CAD build for the part. Positions are in the model's coordinates, mm. Give positions to 0.01 mm unless a question says otherwise; leave off trailing zeros. Loops run counter-clockwise (first coordinate to the right, second up) from the corner with the lowest first, then second, coordinate; pieces in that order, holes last. Notation, with made-up numbers: (69.5, 38) -> (95.5, 38) arc R33 cw to (95.5, 75) -> close; hole circle Ø4 at (8.25, 86). An arc over 180 degrees is marked (long way). Use one line per item in the form item = value.
```python
from build123d import *

# Parameters (mm, degrees)
SKETCH2_R                 = 86.5
SKETCH2_R_2               = 61.5
SKETCH2_R_3               = 2
BOSS_EXTRUDE1_DEPTH       = 5.8
SKETCH3_R                 = 70
SKETCH3_R_2               = 61.5
CUT_EXTRUDE1_DEPTH        = 3
ADVANCEDHOLE1_START       = 3.3
ADVANCEDHOLE1_OUTLINE_R   = 3.925
ADVANCEDHOLE1_OUTLINE_R_2 = 2
ADVANCEDHOLE1_DEPTH       = 2.5
CIRPATTERN1_COUNT         = 6


# Read off the part's stored shape, not the designer's step: AdvancedHole1
with BuildPart() as part:
    # Sketch2 → Boss-Extrude1 (new body)
    with BuildSketch(Plane(origin=(0, 0, 0), x_dir=(1, 0, 0), z_dir=(0, 1, 0))):
        with Locations(Location((0, 0, 0), (0, 0, 270))):
            Circle(SKETCH2_R)
        with Locations(Location((0, 0, 0), (0, 0, 270))):
            Circle(SKETCH2_R_2, mode=Mode.SUBTRACT)
        with Locations(Location((0, 77.5, 0), (0, 0, 270))):
            Circle(SKETCH2_R_3, mode=Mode.SUBTRACT)
        with Locations(Location((67.116968793, 38.75, 0), (0, 0, 270))):
            Circle(SKETCH2_R_3, mode=Mode.SUBTRACT)
        with Locations(Location((67.116968793, -38.75, 0), (0, 0, 270))):
            Circle(SKETCH2_R_3, mode=Mode.SUBTRACT)
        with Locations(Location((0, -77.5, 0), (0, 0, 270))):
            Circle(SKETCH2_R_3, mode=Mode.SUBTRACT)
        with Locations(Location((-67.116968793, -38.75, 0), (0, 0, 270))):
            Circle(SKETCH2_R_3, mode=Mode.SUBTRACT)
        with Locations(Location((-67.116968793, 38.75, 0), (0, 0, 270))):
            Circle(SKETCH2_R_3, mode=Mode.SUBTRACT)
    extrude(amount=BOSS_EXTRUDE1_DEPTH)

    # Sketch3 → Cut-Extrude1 (cut)
    with BuildSketch(Plane.XZ):
        with Locations(Location((0, 0, 0), (0, 0, 270))):
            Circle(SKETCH3_R)
        with Locations(Location((0, 0, 0), (0, 0, 270))):
            Circle(SKETCH3_R_2, mode=Mode.SUBTRACT)
    extrude(amount=-CUT_EXTRUDE1_DEPTH, mode=Mode.SUBTRACT)

    # AdvancedHole1 outline → AdvancedHole1 (cut)
    with BuildSketch(Plane(origin=(0, 0, 0), x_dir=(1, 0, 0), z_dir=(0, 1, 0)).offset(ADVANCEDHOLE1_START)):
        with Locations((-67.116968793, -38.75)):
            Circle(ADVANCEDHOLE1_OUTLINE_R)
        with Locations((-67.116968793, -38.75)):
            Circle(ADVANCEDHOLE1_OUTLINE_R_2, mode=Mode.SUBTRACT)
    advancedhole1 = extrude(amount=ADVANCEDHOLE1_DEPTH, mode=Mode.SUBTRACT)

    # CirPattern1: AdvancedHole1 ×6 about axis
    cirpattern1_axis = Axis((0, 0, 0), (0, 1, 0))
    for i in range(1, CIRPATTERN1_COUNT):
        add(advancedhole1.rotate(cirpattern1_axis, i * 360 / CIRPATTERN1_COUNT), mode=Mode.SUBTRACT)


solid = part.part
```
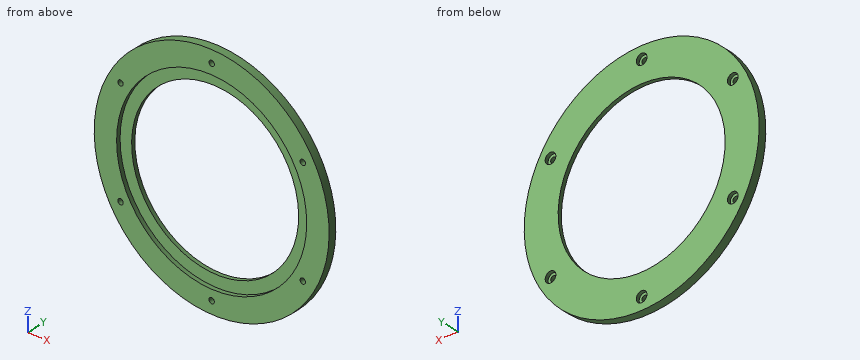
1. Cut at D-D, the plane x = 34.5. Write the cut outline in (y, z), then the cut area to 3 significant figures.
Result sheet:
outline = (0, -79.32) -> (5.8, -79.32) -> (5.8, -50.91) -> (3, -50.91) -> (3, -60.91) -> (0, -60.91) -> close; (0, 60.91) -> (3, 60.91) -> (3, 50.91) -> (5.8, 50.91) -> (5.8, 79.32) -> (0, 79.32) -> close
area = 270 mm^2
2. Cut at C-C, the plane y = 1.85. Write the cut outline in (x, z).
Result sheet:
outline = circle Ø173 at (0, 0); hole circle Ø140 at (0, 0); hole circle Ø4 at (-67.12, -38.75); hole circle Ø4 at (-67.12, 38.75); hole circle Ø4 at (0, -77.5); hole circle Ø4 at (0, 77.5); hole circle Ø4 at (67.12, -38.75); hole circle Ø4 at (67.12, 38.75)
3. Cut at A-A, the plane z = 0. Write the cut outline in (x, y), then the cut area to 3 significant figures.
Result sheet:
outline = (-86.5, 0) -> (-70, 0) -> (-70, 3) -> (-61.5, 3) -> (-61.5, 5.8) -> (-86.5, 5.8) -> close; (61.5, 3) -> (70, 3) -> (70, 0) -> (86.5, 0) -> (86.5, 5.8) -> (61.5, 5.8) -> close
area = 239 mm^2
4. Drill centre lines: line 1 (Z direction, x = 0.5, y = 3.55); line 2 (X direction, y = 4.9, z = 38.75); line 3 (X direction, y = 2.5, z = -38.75). Where is each one in solid material? Low to high.
Result sheet:
line_1 = -86.5 to -81.39, -73.61 to -61.5, 61.5 to 73.61, 81.39 to 86.5
line_2 = -77.33 to -71.04, -63.19 to -47.76, 47.76 to 63.19, 71.04 to 77.33
line_3 = -77.33 to -69.12, -65.12 to -58.3, 58.3 to 65.12, 69.12 to 77.33
5. Drop flat-ended pins along their axis: P1, Ø10, axis at x = 0, z = -77.5, coming from the -Y side; P2, Ø2.5, axis at x = -68.5, z = -39, coming from the +Y side; P3, Ø1, axis at x = -60.5, y = 4.5, coming from the +Z side; P4, Ø2, axis at y = 0.5, z = -44.5, coming from the +X side. Give the stop position or say it passes through.
Result sheet:
P1 = 0
P2 = 3.3
P3 = 62.31
P4 = 74.77
6. Cut at B-B, the plane x = 0. Write the cut outline in (y, z) (3 decimals), then the cut area to 3 significant figures.
Result sheet:
outline = (0, -86.5) -> (5.8, -86.5) -> (5.8, -81.425) -> (3.3, -81.425) -> (3.3, -79.5) -> (0, -79.5) -> close; (0, -75.5) -> (3.3, -75.5) -> (3.3, -73.575) -> (5.8, -73.575) -> (5.8, -61.5) -> (3, -61.5) -> (3, -70) -> (0, -70) -> close; (0, 70) -> (3, 70) -> (3, 61.5) -> (5.8, 61.5) -> (5.8, 73.575) -> (3.3, 73.575) -> (3.3, 75.5) -> (0, 75.5) -> close; (0, 79.5) -> (3.3, 79.5) -> (3.3, 81.425) -> (5.8, 81.425) -> (5.8, 86.5) -> (0, 86.5) -> close
area = 173 mm^2
